The model under review builds one solid part; all positions refer to its coordinate system, in mm. Give positions to 0.01 mm unless a question says otherwise; leave off trailing zeros. Order: outer loops, then holes, each group sorted by start corner. A loop starts at its lowest first (then second) coordinate and runs counter-clockwise, first axis right, second up.
```python
from build123d import *

# Parameters (mm, degrees)
F1_DEPTH = 1
F2_R     = 10
F3_DEPTH = 1.001


with BuildPart() as f1:
    # F0 (on Front) → F1 (new body)
    with BuildSketch(Plane.XZ):
        Polygon((-107.687899, 590.256992), (0, 0), (1623.206728, 296.141721), (708.831554, 2024.061715), align=None)
    extrude(amount=F1_DEPTH)

    # F2 (on face) → F3 (cut, through all)
    with BuildSketch(Plane.XZ.offset(1)):
        with Locations((-76.215289, 584.899588)):
            Circle(F2_R)
        with Locations((185.070935, 1043.717099)):
            Circle(F2_R)
        with Locations((446.35716, 1502.534611)):
            Circle(F2_R)
        with Locations((707.643385, 1961.352122)):
            Circle(F2_R)
        with Locations((24.128455, 34.897245)):
            Circle(F2_R)
        with Locations((1577.53703, 318.304824)):
            Circle(F2_R)
    extrude(amount=-F3_DEPTH, mode=Mode.SUBTRACT)


solid = f1.part
```
Item 1: Take a section at C-C (x = 814.5). Give the boundary of the cut face in (y, z), and give its area (3 significant figures).
Values found:
outline: (-1, 148.6) - (0, 148.6) - (0, 1824.38) - (-1, 1824.38) - close
area: 1,680 mm2
Item 2: Take a section at A-A (y = -0.45). Give the boundary of the cut face in (x, z), and give its area (3 significant figures).
Values found:
outline: (-107.69, 590.26) - (0, 0) - (1623.21, 296.14) - (708.83, 2024.06) - close; hole circle Ø20 at (-76.22, 584.9); hole circle Ø20 at (24.13, 34.9); hole circle Ø20 at (185.07, 1043.72); hole circle Ø20 at (446.36, 1502.53); hole circle Ø20 at (707.64, 1961.35); hole circle Ø20 at (1577.54, 318.3)
area: 1,850,000 mm2
Item 3: For line 1 (X direction, y = -0.2, z = 320); line 2 (Z direction, x = 759.5, y = -0.25) (3 decimals); line 3 (X direction, y = -0.8, z = 313), list the stretches that pass through material, from the lowest coordinate up.
Values found:
line 1: x = -58.38 to 1567.68, 1587.39 to 1610.58
line 2: z = 138.565 to 1928.312
line 3: x = -57.1 to 1569.06, 1586.01 to 1614.29
Item 4: Take a section at B-B (z = 227). Give the boundary of the cut face in (x, y).
Values found:
outline: (-41.41, -1) - (1244.23, -1) - (1244.23, 0) - (-41.41, 0) - close
